from build123d import *

# Parameters (mm, degrees)
BASPROSKE_W         = 6
BASPROSKE_H         = 12.75
TOOTHCUT_DEPTH      = 20.003289189
TEETHCUTS_COUNT     = 15
TEETHCUTS_ANGLE     = 336
BORSKE_R            = 3
BORE_DEPTH          = 50.0000508
BOSS_EXTRUDE1_START = 7
SKETCH1_R           = 5
SKETCH1_R_2         = 3
BOSS_EXTRUDE1_DEPTH = 7
CUT_EXTRUDE1_START  = -7
CUT_EXTRUDE1_DEPTH  = 7
SKETCH3_W           = 7
SKETCH3_H           = 5.292923502
BOSS_EXTRUDE2_DEPTH = 1.5


# Read off the part's stored shape, not the designer's step: Cut-Extrude1
with BuildPart() as part:
    # BasProSke → Base-Revolve (revolve)
    with BuildSketch(Plane(origin=(0, 0, 0), x_dir=(1, 0, 0), z_dir=(0, 1, 0)), mode=Mode.PRIVATE) as base_revolve_sk:
        with Locations((3, 6.375)):
            Rectangle(BASPROSKE_W, BASPROSKE_H)
    revolve(base_revolve_sk.sketch.rotate(Axis((-10, 0, 0), (1, 0, 0)), 180), axis=Axis((-10, 0, 0), (1, 0, 0)))

    # TooCutSke → ToothCut (cut, through all)
    with BuildSketch(Plane(origin=(0, 0, 0), x_dir=(0, 0, -1), z_dir=(1, 0, 0))):
        with BuildLine():
            ThreePointArc((0.791546546, 9.340520867), (0, 9.374), (-0.791546546, 9.340520867))
            ThreePointArc((-0.791546546, 9.340520867), (-1.235070734, 11.110218102), (-2.344732916, 12.558386549))
            ThreePointArc((-2.344732916, 12.558386549), (0, 12.7754), (2.344732916, 12.558386549))
            ThreePointArc((2.344732916, 12.558386549), (1.235070734, 11.110218102), (0.791546546, 9.340520867))
        make_face()
    toothcut = extrude(amount=TOOTHCUT_DEPTH, mode=Mode.SUBTRACT)

    # TeethCuts: ToothCut ×15 about axis
    teethcuts_axis = Axis((-10, 0, 0), (1, 0, 0))
    for i in range(1, TEETHCUTS_COUNT):
        add(toothcut.rotate(teethcuts_axis, i * TEETHCUTS_ANGLE / (TEETHCUTS_COUNT - 1)), mode=Mode.SUBTRACT)

    # BorSke → Bore (cut, symmetric)
    with BuildSketch(Plane(origin=(0, 0, 0), x_dir=(0, 0, -1), z_dir=(1, 0, 0))):
        with Locations(Location((0, 0, 0), (0, 0, 180))):
            Circle(BORSKE_R)
    extrude(amount=BORE_DEPTH, both=True, mode=Mode.SUBTRACT)

    # Sketch1 → Boss-Extrude1 (add)
    with BuildSketch(Plane(origin=(6, 0, 0), x_dir=(0, 0, -1), z_dir=(1, 0, 0)).offset(BOSS_EXTRUDE1_START)):
        with Locations(Location((0, 0, 0), (0, 0, 180))):
            Circle(SKETCH1_R)
        Circle(SKETCH1_R_2, mode=Mode.SUBTRACT)
    extrude(amount=-BOSS_EXTRUDE1_DEPTH)

    # Cut-Extrude1 outline → Cut-Extrude1 (cut)
    with BuildSketch(Plane(origin=(13, 0, 0), x_dir=(0, 0, -1), z_dir=(1, 0, 0)).offset(CUT_EXTRUDE1_START)):
        with BuildLine():
            ThreePointArc((2.869678463, 0.874611639), (2.997049903, -0.133010816), (2.780917301, -1.125388361))
            Line((2.780917301, -1.125388361), (4.87170412, -1.125388361))
            ThreePointArc((4.87170412, -1.125388361), (4.998361954, -0.127975708), (4.922911179, 0.874611639))
            Line((4.922911179, 0.874611639), (2.869678463, 0.874611639))
        make_face()
    extrude(amount=CUT_EXTRUDE1_DEPTH, mode=Mode.SUBTRACT)

    # Sketch3 → Boss-Extrude2 (add)
    with BuildSketch(Plane(origin=(0, -1.125388361, 0), x_dir=(1, 0, 0), z_dir=(0, 1, 0))):
        with Locations((9.5, 5.427379052)):
            Rectangle(SKETCH3_W, SKETCH3_H)
    boss_extrude2 = extrude(amount=-BOSS_EXTRUDE2_DEPTH)

    # Mirror2: Boss-Extrude2 across plane
    add(boss_extrude2.mirror(Plane.ZX))


solid = part.part
Here's how the part is built. I have some questions about the finished solid (model axes, mm). A direction names the side the tool comes from. Coordinates: 2 decimals unless noted, no trailing zeros. Write each loop counter-clockwise with the first axis right and the second up, starting at its lowest first coordinate (ties: lowest second). Pieces come first, ordered by that corner, then holes.
1) If we section it at C-C (z = 4): List the corners of the cut face in (x, y) for me, plus the area to 3 significant figures.
Filled in:
outline: (0, -11.14) - (6, -11.14) - (6, -3) - (13, -3) - (13, 3) - (6, 3) - (6, 8.48) - (0, 8.48) - close
area: 160 mm2
2) If we section it at A-A (z = 0): List the corners of the cut face in (x, y) for me, plus the area to 3 significant figures.
Filled in:
outline: (0, -12.75) - (6, -12.75) - (6, -5) - (13, -5) - (13, -3) - (0, -3) - close; (0, 3) - (13, 3) - (13, 5) - (6, 5) - (6, 9.37) - (0, 9.37) - close
area: 125 mm2
3) I'm going to push flat-ended pins straight in: pin 1 (1.5 mm diameter, centred on x = 4.5, z = 9, fed in from +Y); pin 2 (3.5 mm diameter, centred on y = 0, z = 0, fed in from +X); pin 3 (1.6 mm diameter, centred on x = 10, y = 1.5, fed in from -Z); pin 4 (1.9 mm diameter, centred on x = 9.5, z = -5.5, fed in from -Y). Where does each tip first touch, or does it pass through?
Filled in:
pin 1: stops at y = 6.66
pin 2: passes through
pin 3: stops at z = -8.07
pin 4: stops at y = -2.63
4) If we section it at B-B (x = 7): List the corners of the cut face in (y, z) for me.
Filled in:
outline: (-2.63, -8.07) - (-1.13, -8.07) - (-1.13, -2.78) arc R3 cw (long way) to (0.87, -2.87) - (0.87, -4.92) arc R5 ccw to (1.13, -4.87) - (1.13, -8.07) - (2.63, -8.07) - (2.63, -4.26) arc R5 ccw (long way) to (-2.63, -4.26) - close
5) If I drill on line 1 (Y direction, x = 9, z = 0); line 2 (Z direction, x = 5.75, y = -9.5); line 3 (Z direction, x = 10.25, y = 0), over which ranges is the centre line in solid material (lowest first)?
Filled in:
line 1: y = -5 to -3, 3 to 5
line 2: z = -5.49 to -2.89, -1.2 to 1.2, 2.89 to 5.49
line 3: z = 3 to 5
6) Thinking about a two-plate mould opening in Z: for faces 1 (the face through (2.96, -6.63, -9.01)), 2 (the face through (9, 2.625, -6)), 3 (the face through (2.96, 8.56, -3.82)), which applies, +Z half, -Z half, draft (parallel to the pull), parting line (faces both ways), or undercut?
Filled in:
face 1: -Z half
face 2: draft
face 3: undercut
7) Which directions (+Z, -Z, +X, -X, +Y, -Y) give clear straight access to the entire face, cutting with the end or side of a thin tool? Please do faces 4 (the face through (9, -2.625, -6)), 5 (the face through (2.958, -10.618, 3.524)), 6 (the face through (2.958, 8.361, 7.434)), 7 (the face through (10, 0, 5)), 8 (the face through (2.96, 10.66, 3.39)).
Filled in:
face 4: -Z, +X, -Y
face 5: +X, -X, -Y
face 6: +Z, +X, -X
face 7: +X
face 8: +X, -X
